The model under review builds one solid part; all positions refer to its coordinate system, in mm. Face numbers are marked on the shaded views. A direction names the side the tool comes from. Round coordinates to 2 decimals unless told otherwise and drop trailing zeros. Loops run counter-clockwise (first coordinate to the right, second up) from the corner with the lowest first, then second, coordinate; pieces in that order, holes last. Notation, with made-up numbers: M 62.25,7 L 85.25,7 A23 ccw 85.25,43 Z; hole C 0.25,10.5 d2. An arc over 180 degrees is marked long. Use a Markdown table: item, result. Add a question column.
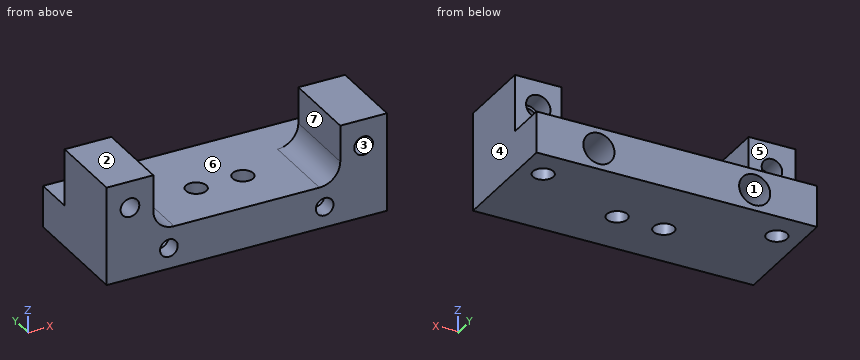
```python
from build123d import *

# Parameters (mm, degrees)
SKETCH1_W                                    = 38
SKETCH1_H                                    = 8
BOSS_EXTRUDE1_DEPTH                          = 22.75
SKETCH9_W                                    = 9
SKETCH9_H                                    = 5
BOSS_EXTRUDE2_DEPTH                          = 19
SKETCH8_R                                    = 3
CUT_EXTRUDE1_DEPTH                           = 18
CSK_FOR_M3_COUNTERSUNK_FLAT_HEAD_SCR_2_COUNT = 2
CSK_FOR_M3_COUNTERSUNK_FLAT_HEAD_SCR_2_PITCH = 30
FILLET1_R                                    = 2
BOSS_EXTRUDE3_DEPTH                          = 22.75
SKETCH16_R                                   = 1.98
CUT_EXTRUDE4_DEPTH                           = 8
SKETCH14_W                                   = 54
SKETCH14_H                                   = 11
CUT_EXTRUDE6_DEPTH                           = 7.75
SKETCH15_R                                   = 1.98
SKETCH15_R_2                                 = 2.35
CUT_EXTRUDE7_DEPTH                           = 4
M3_CLEARANCE_HOLE2_D                         = 3.6
FILLET2_R                                    = 4


with BuildPart() as part:
    # Sketch1 → Boss-Extrude1 (new body)
    with BuildSketch(Plane(origin=(0, 0, 0), x_dir=(1, 0, 0), z_dir=(0, 1, 0))):
        Rectangle(SKETCH1_W, SKETCH1_H)
    extrude(amount=BOSS_EXTRUDE1_DEPTH)

    # Sketch9 → Boss-Extrude2 (add)
    with BuildSketch(Plane.XY.offset(-4)):
        with Locations((-22.5, 12.5)):
            Rectangle(SKETCH9_W, SKETCH9_H)
        with Locations((22.5, 12.5)):
            Rectangle(SKETCH9_W, SKETCH9_H)
    extrude(amount=BOSS_EXTRUDE2_DEPTH)

    # Sketch8 → Cut-Extrude1 (cut)
    with BuildSketch(Plane(origin=(0, 22.75, 0), x_dir=(1, 0, 0), z_dir=(0, 1, 0))):
        with Locations(Location((-15, 0, 0), (0, 0, 270))):
            Circle(SKETCH8_R)
        with Locations(Location((15, 0, 0), (0, 0, 270))):
            Circle(SKETCH8_R)
    extrude(amount=-CUT_EXTRUDE1_DEPTH, mode=Mode.SUBTRACT)

    # Sketch4 → CSK for M3 Countersunk Flat Head Screw1 (revolve, cut)
    with BuildSketch(Plane(origin=(-15, 4.75, 0), x_dir=(0, 0, 1), z_dir=(1, 0, 0))):
        Polygon((0, 0), (0, 4.75), (1.7, 4.75), (1.7, 1.45), (3.15, 0), align=None)
    csk_for_m3_countersunk_flat_head_screw1 = revolve(axis=Axis((-15, 11.1, 0), (0, -1, 0)), mode=Mode.SUBTRACT)

    # CSK for M3 Countersunk Flat Head Scr 2: CSK for M3 Countersunk Flat Head Screw1 ×2
    with Locations(*[(i * CSK_FOR_M3_COUNTERSUNK_FLAT_HEAD_SCR_2_PITCH, 0, 0) for i in range(1, CSK_FOR_M3_COUNTERSUNK_FLAT_HEAD_SCR_2_COUNT)]):
        add(csk_for_m3_countersunk_flat_head_screw1, mode=Mode.SUBTRACT)

    # Fillet1
    fillet1_edges = [part.edges().sort_by_distance(p)[0] for p in [
        (-27, 12.5, 15),
        (-18, 12.5, 15),
        (27, 12.5, 15),
        (18, 12.5, 15),
    ]]
    fillet(fillet1_edges, radius=FILLET1_R)

    # Sketch13 → Boss-Extrude3 (add)
    with BuildSketch(Plane(origin=(0, 0, 0), x_dir=(-1, 0, 0), z_dir=(0, -1, 0))):
        Polygon((-18, -4), (-18, 4), (-27, 4), (-27, -4), (-27, -15), (-18, -15), align=None)
        Polygon((27, 4), (18, 4), (18, -4), (18, -15), (27, -15), (27, -4), align=None)
    extrude(amount=-BOSS_EXTRUDE3_DEPTH)

    # Sketch16 → Cut-Extrude4 (cut)
    with BuildSketch(Plane.XY.offset(-4)):
        with Locations((-22.5, 16.75)):
            Circle(SKETCH16_R)
        with Locations((-4.5, 9.75)):
            Circle(SKETCH16_R)
        with Locations((4.5, 9.75)):
            Circle(SKETCH16_R)
        with Locations((22.5, 16.75)):
            Circle(SKETCH16_R)
    extrude(amount=CUT_EXTRUDE4_DEPTH, mode=Mode.SUBTRACT)

    # Sketch14 → Cut-Extrude6 (cut)
    with BuildSketch(Plane(origin=(0, 22.75, 0), x_dir=(1, 0, 0), z_dir=(0, 1, 0))):
        with Locations((0, -9.5)):
            Rectangle(SKETCH14_W, SKETCH14_H)
    extrude(amount=-CUT_EXTRUDE6_DEPTH, mode=Mode.SUBTRACT)

    # Sketch15 → Cut-Extrude7 (cut)
    with BuildSketch(Plane(origin=(0, 15, 0), x_dir=(1, 0, 0), z_dir=(0, 1, 0))):
        with Locations(Location((-22.5, -9.9, 0), (0, 0, 270))):
            Circle(SKETCH15_R)
        with Locations(Location((22.5, -9.9, 0), (0, 0, 270))):
            Circle(SKETCH15_R_2)
    extrude(amount=-CUT_EXTRUDE7_DEPTH, mode=Mode.SUBTRACT)

    # M3 Clearance Hole2 (through all)
    with Locations(Plane(origin=(0, 11, 0), x_dir=(1, 0, 0), z_dir=(0, 1, 0))):
        with Locations((-22.5, -9.9), (22.5, -9.9)):
            Hole(M3_CLEARANCE_HOLE2_D / 2)

    # Fillet2
    fillet2_edges = [part.edges().sort_by_distance(p)[0] for p in [
        (-18, 7.5, 4),
        (18, 7.5, 4),
    ]]
    fillet(fillet2_edges, radius=FILLET2_R)


solid = part.part
```
(1) Draft analysis for pull direction Z (two halves, no side actions). For the marked faces 1, 2, 3 and 4, state which applies: released by +Z, released by -Z, zero draft, split by the parting line, or undercut.
(2) Consider section D-D, the plane z = 14. Give the boundary of the cut face in (x, y), then the cut area to 3 significant figures.
(3) Consider section C-C, the plane y = 12.75. Give the boundary of the cut face in (x, z), then the cut area to 3 significant figures.
(4) Consider section A-A, the plane y = 16.75. Give the boundary of the cut face in (x, z), then the cut area to 3 significant figures.
(5) Insertion check: pin 1 Ø4 at (x, z) = (22.5, 9.9) entering from +Y; pin 2 Ø2 at (x, y) = (17, 20) entering from +Z; pin 3 Ø4.5 at (x, z) = (-22.5, 9) entering from +Y; pin 4 Ø3 at (x, z) = (-22.5, 9.9) entering from -Y. Each pin has a flat end and moves straight along its axis. Give the tip position at first contact, or say it passes through.
(6) Consider section B-B, the plane z = 9.9. Give the boundary of the cut face in (x, y), then the cut area to 3 significant figures.
(7) For the marked faces 5, 6 and 7, list the 3-axis set-ups (+Z, -Z, +X, -X, +Y, -Y) from which the entire face can be reached by the end or side of a thin tool; tool diameter is ignored.
(8) To check wall thickness, follow probe 1 along X at (y, z) = (2.6, 0); probe 2 along X at (y, z) = (7.5, 9.9); probe 3 along X at (y, z) = (12.8, 9.9). State the ranges of each line that lie inside material, in increasing order.
Found:
| question | item | result |
|---|---|---|
| 1 | face 1 | undercut |
| 1 | face 2 | released by +Z |
| 1 | face 3 | undercut |
| 1 | face 4 | zero draft |
| 2 | outline | M -27,0 L -18,0 L -18,15 L -27,15 Z; M 18,0 L 27,0 L 27,15 L 18,15 Z |
| 2 | area | 270 mm^2 |
| 3 | outline | M -27,-4 L 27,-4 L 27,15 L 18,15 L 18,8 A4 cw 14,4 L -14,4 A4 cw -18,8 L -18,15 L -27,15 Z; hole C -22.5,9.9 d3.96; hole C -15,0 d6; hole C 15,0 d6; hole C 22.5,9.9 d4.7 |
| 3 | area | 551 mm^2 |
| 4 | outline | M -27,-4 L -24.48,-4 L -24.48,4 L -27,4 Z; M -20.52,-4 L 20.52,-4 L 20.52,4 L -20.52,4 Z; M 24.48,-4 L 27,-4 L 27,4 L 24.48,4 Z; hole C -15,0 d6; hole C 15,0 d6 |
| 4 | area | 312 mm^2 |
| 5 | pin 1 | stops at y = 11 |
| 5 | pin 2 | stops at z = 4 |
| 5 | pin 3 | stops at y = 15 |
| 5 | pin 4 | passes through |
| 6 | outline | M -27,0 L -24.3,0 L -24.3,11 L -24.48,11 L -24.48,15 L -27,15 Z; M -20.7,0 L -18,0 L -18,15 L -20.52,15 L -20.52,11 L -20.7,11 Z; M 18,0 L 20.7,0 L 20.7,11 L 20.15,11 L 20.15,15 L 18,15 Z; M 24.3,0 L 27,0 L 27,15 L 24.85,15 L 24.85,11 L 24.3,11 Z |
| 6 | area | 156 mm^2 |
| 7 | face 5 | +Z, +X, -X, +Y |
| 7 | face 6 | +Z, +Y |
| 7 | face 7 | +Z, +Y, -Y |
| 8 | probe 1 | x = -27 to -16.7, -13.3 to 13.3, 16.7 to 27 |
| 8 | probe 2 | x = -27 to -24.3, -20.7 to -18, 18 to 20.7, 24.3 to 27 |
| 8 | probe 3 | x = -27 to -24.48, -20.52 to -18, 18 to 20.15, 24.85 to 27 |
